```python
from build123d import *

# Parameters (mm, degrees)
SKETCH1_R                   = 20
BOSS_EXTRUDE1_DEPTH         = 7
TAP_DRILL_FOR_M6X1_0_TAP1_D = 5
CIRPATTERN1_COUNT           = 6
SKETCH3_R                   = 6.35
BOSS_EXTRUDE2_DEPTH         = 70


with BuildPart() as part:
    # Sketch1 → Boss-Extrude1 (new body)
    with BuildSketch(Plane.XY):
        Circle(SKETCH1_R)
    extrude(amount=BOSS_EXTRUDE1_DEPTH)

    # Tap Drill for M6x1.0 Tap1 (through all)
    with Locations(Plane.XY.offset(7)):
        with Locations((0, 12.5)):
            tap_drill_for_m6x1_0_tap1 = Hole(TAP_DRILL_FOR_M6X1_0_TAP1_D / 2)

    # CirPattern1: Tap Drill for M6x1.0 Tap1 ×6 about axis
    cirpattern1_axis = Axis((0, 0, 0), (0, 0, 1))
    for i in range(1, CIRPATTERN1_COUNT):
        add(tap_drill_for_m6x1_0_tap1.rotate(cirpattern1_axis, i * 360 / CIRPATTERN1_COUNT), mode=Mode.SUBTRACT)

    # Sketch3 → Boss-Extrude2 (add)
    with BuildSketch(Plane.XY.offset(7)):
        Circle(SKETCH3_R)
    extrude(amount=BOSS_EXTRUDE2_DEPTH)


solid = part.part
```
Design review of the part built by this model. Coordinates are the model's own, in mm. Round coordinates to 2 decimals unless told otherwise and drop trailing zeros. Write each loop counter-clockwise with the first axis right and the second up, starting at its lowest first coordinate (ties: lowest second). Pieces come first, ordered by that corner, then holes. Notation, with made-up numbers: (8, 5) -> (40, 5) arc R9 cw to (40, 22) -> close; hole circle Ø11 at (83.5, 28.25). An arc over 180 degrees is marked (long way). Write item = value, one per line. Start each with the question number.
1) Take a section at D-D, the plane z = 34. State the section outline as (x, y) points.
2) Clearance check with flat-ended pins moving along their axes: pin 1 (4 mm diameter, centred on x = -10.83, y = -6.25, fed in from +Z); pin 2 (8 mm diameter, centred on x = 10, y = -14, fed in from +Z); pin 3 (8 mm diameter, centred on y = 6.5, z = 41, fed in from +X); pin 4 (4 mm diameter, centred on y = -7.5, z = 41.5, fed in from +X). State where each tip first meets the part, or that it passes through.
3) Take a section at C-C, the plane y = 0. State the section outline as (x, z) points, plus the area to 3 significant figures.
4) Take a section at A-A, the plane x = 0. State the section outline as (y, z) points.
5) Take a section at B-B, the plane y = -12.5. State the section outline as (x, z) points.
6) Wall thickness on probe 1 along Y at (x, z) = (0, 5); probe 2 along X at (y, z) = (-7.5, 5.5); probe 3 along Z at (x, y) = (-3, -7.5): over which ranges is each line inside the solid? List them lowest first. Write a range as from..to.
7) Mouldability with a two-part tool opening along Y and no side actions: class faces 1 (the face through (-1.38, -6.2, 41.51)), 2 (the face through (-5, 5, 7)), 3 (the face through (-0.54, -10.06, 3.45)) as +Y half, -Y half, draft (parallel to the pull), parting line (faces both ways), or undercut.
Results list:
q1.outline = circle Ø12.7 at (0, 0)
q2.pin_1 = through
q2.pin_2 = 7
q2.pin_3 = 5.84
q2.pin_4 = 3.17
q3.outline = (-20, 0) -> (20, 0) -> (20, 7) -> (6.35, 7) -> (6.35, 77) -> (-6.35, 77) -> (-6.35, 7) -> (-20, 7) -> close
q3.area = 1,170 mm²
q4.outline = (-20, 0) -> (-15, 0) -> (-15, 7) -> (-20, 7) -> close; (-10, 0) -> (10, 0) -> (10, 7) -> (6.35, 7) -> (6.35, 77) -> (-6.35, 77) -> (-6.35, 7) -> (-10, 7) -> close; (15, 0) -> (20, 0) -> (20, 7) -> (15, 7) -> close
q5.outline = (-15.61, 0) -> (-2.5, 0) -> (-2.5, 7) -> (-15.61, 7) -> close; (2.5, 0) -> (15.61, 0) -> (15.61, 7) -> (2.5, 7) -> close
q6.probe_1 = -20..-15, -10..10, 15..20
q6.probe_2 = -18.54..-12.99, -8.66..8.66, 12.99..18.54
q6.probe_3 = 0..7
q7.face_1 = parting line
q7.face_2 = draft
q7.face_3 = undercut
